Verification items for the finished model (mm, model axes). Coordinates: 2 decimals unless noted, no trailing zeros. Order: outer loops, then holes, each group sorted by start corner. A loop starts at its lowest first (then second) coordinate and runs counter-clockwise, first axis right, second up. Notation, with made-up numbers: (-33.75, -13) - (19.25, -13) arc R22 ccw to (19.25, 10) - close; hole circle Ø5 at (23.5, 13.5). An arc over 180 degrees is marked (long way). Answer as CSV lines item,"result". Start each with the question number.
1. Section check A-A (x = 0). Record the cut outline in (y, z), and give its area (3 significant figures).
2. Go/stop test with flat-tipped pins: pin 1 (1 mm diameter, centred on y = -26, z = -14, fed in from +X); pin 2 (3 mm diameter, centred on y = -11.5, z = -28.5, fed in from -X); pin 3 (2 mm diameter, centred on x = 18.5, z = -30, fed in from +Y). Record where each tip stops, or that it passes through.
3. Material ranges on L1, parallel to Y at x = -26, z = -15; L2, parallel to Y at x = -17, z = -36; L3, parallel to X at y = 7.5, z = -15, recorded low to high. Write a range as [from, to].
4. Section check C-C (z = -13.5). Record the cut outline in (x, y).
from build123d import *

# Parameters (mm, degrees)
SKETCH1_R           = 50
BOSS_EXTRUDE1_DEPTH = 5
REVOLVE1_ANGLE      = 180


with BuildPart() as part:
    # Sketch1 → Boss-Extrude1 (new body)
    with BuildSketch(Plane.XY):
        Circle(SKETCH1_R)
    extrude(amount=-BOSS_EXTRUDE1_DEPTH)

    # Sketch2 → Revolve1 (revolve)
    with BuildSketch(Plane(origin=(0, 0, -5), x_dir=(-1, 0, 0), z_dir=(0, 0, -1))):
        with BuildLine():
            Line((0, -50), (0, 50))
            ThreePointArc((0, 50), (50, 0), (0, -50))
        make_face()
    revolve(axis=Axis((0, -50, -5), (0, -1, 0)), revolution_arc=REVOLVE1_ANGLE)

    # Sketch4 → Cut-Revolve1 (revolve, cut)
    with BuildSketch(Plane.XY):
        with BuildLine():
            Line((0, -46), (0, 46))
            ThreePointArc((0, 46), (46, 0), (0, -46))
        make_face()
    revolve(axis=Axis((0, -46, 0), (0, 1, 0)), mode=Mode.SUBTRACT)


solid = part.part
Evaluation:
1,outline,"(-50, -5) arc R50 ccw to (50, -5) - (50, 0) - (46, 0) arc R46 cw to (-46, 0) - (-50, 0) - close"
1,area,"1,100 mm²"
2,pin 1,"stops at x = 42.07"
2,pin 2,"stops at x = -43.49"
2,pin 3,"stops at y = 39.92"
3,L1,"y = [-41.52, -34.86], [34.86, 41.52]"
3,L2,"y = [-35.36, -23.04], [23.04, 35.36]"
3,L3,"x = [-48.41, -42.83], [42.83, 48.41]"
4,outline,"circle Ø98.54 at (0, 0); hole circle Ø87.95 at (0, 0)"
